```python
from build123d import *

# Parameters (mm, degrees)
F0_W     = 1370
F0_H     = 93
F1_DEPTH = 9
F2_W     = 1370
F2_H     = 75
F3_DEPTH = 9
F4_SIZE  = 10
F5_SIZE  = 5


with BuildPart() as f1:
    # F0 (on Front) → F1 (new body)
    with BuildSketch(Plane.XZ):
        Rectangle(F0_W, F0_H)
    extrude(amount=F1_DEPTH)

    # F2 (on face) → F3 (join)
    with BuildSketch(Plane.XZ.offset(9)):
        with Locations((0, 9)):
            Rectangle(F2_W, F2_H)
    extrude(amount=F3_DEPTH)

    # F4
    f4_edges = [f1.edges().sort_by_distance(p)[0] for p in [
        (685, -4.5, -46.5),
        (-685, -4.5, -46.5),
    ]]
    chamfer(f4_edges, length=F4_SIZE)

    # F5
    f5_edges = [f1.edges().sort_by_distance(p)[0] for p in [
        (0, 0, -46.5),
    ]]
    chamfer(f5_edges, length=F5_SIZE)


solid = f1.part
```
Can you work these out from the model? Positions are in its coordinate system, mm. Coordinates: 2 decimals unless noted, no trailing zeros. Loops run counter-clockwise (first coordinate to the right, second up) from the corner with the lowest first, then second, coordinate; pieces in that order, holes last.
1) I need wall thicknesses on probe 1 along Z at (x, y) = (-100.5, -14.75); probe 2 along Z at (x, y) = (560.5, -1); probe 3 along X at (y, z) = (-6, -38.5). Which ranges of each line are inside material? Lowest first, please.
2) For pin 1 (4.5 mm diameter, centred on x = 137.5, y = -13.5, fed in from -Z); pin 2 (9 mm diameter, centred on x = 64.5, z = -37, fed in from -Y), each with a flat end and sliding along its axis, tell me the tip position at first contact or that it passes through.
3) Imagine slicing it at A-A on x = -170. List the corners of the cut face in (y, z) for me, plus the area to 3 significant figures.
4) Imagine slicing it at B-B on y = -12.5. List the corners of the cut face in (x, z) for me, plus the area to 3 significant figures.
Completed:
1. probe 1: z = -28.5 to 46.5
1. probe 2: z = -42.5 to 46.5
1. probe 3: x = -683 to 683
2. pin 1: stops at z = -28.5
2. pin 2: stops at y = -9
3. outline: (-18, -28.5) - (-9, -28.5) - (-9, -46.5) - (-5, -46.5) - (0, -41.5) - (0, 46.5) - (-18, 46.5) - close
3. area: 1,500 mm2
4. outline: (-685, -28.5) - (685, -28.5) - (685, 46.5) - (-685, 46.5) - close
4. area: 103,000 mm2
